Autodesk Inventor part; units mm, degrees
ref_plane "YZ Plane" through (0, 0, 0) normal (1, 0, 0) x (0, 1, 0)
ref_plane "XZ Plane" through (0, 0, 0) normal (0, 1, 0) x (-1, 0, 0)
ref_plane "XY Plane" through (0, 0, 0) normal (0, 0, 1) x (1, 0, 0)
sketch "Sketch1" plane through (0, 0, 0) normal (0, 1, 0) x (-1, 0, 0)
  line L0 (-10, 14) -> (-10, -14)
  line L1 (-7.5, -16.5) -> (7.5, -16.5)
  line L2 (10, -14) -> (10, 14)
  line L3 (7.5, 16.5) -> (-7.5, 16.5)
  line L4 (-10, 16.5) -> (10, -16.5) construction
  line L5 (-10, -16.5) -> (10, 16.5) construction
  arc A0 (10, 14) -> (7.5, 16.5) centre (7.5, 14) ccw
  arc A1 (7.5, -16.5) -> (10, -14) centre (7.5, -14) ccw
  arc A2 (-10, -14) -> (-7.5, -16.5) centre (-7.5, -14) ccw
  arc A3 (-7.5, 16.5) -> (-10, 14) centre (-7.5, 14) ccw
  circle A4 centre (7.5, 14) radius 1.25
  circle A5 centre (-7.5, 14) radius 1.25
  circle A6 centre (-7.5, -14) radius 1.25
  circle A7 centre (7.5, -14) radius 1.25
  point P0 (0, 0)
  dimension "d0" = 33
  dimension "d1" = 20
  dimension "d2" = 2.5
  dimension "d3" = 2.5
  dimension "d4" = 2.5
  dimension "d5" = 2.5
  dimension "d6" = 2.5
extrude "Extrusion1" add sketch "Sketch1" along normal blind 2
sketch "Sketch2" plane through (0, 2, 0) normal (0, 1, 0) x (1, 0, 0)
  line L0 (-17.9692, -32.7187) -> (-17.5216, 33.3599) construction
  line L1 (-17.5216, 33.3599) -> (32.0714, 33.0239) construction
  line L2 (32.0714, 33.0239) -> (31.6238, -33.0546) construction
  line L3 (31.6238, -33.0546) -> (-17.9692, -32.7187) construction
  circle A0 centre (-7.5, 14) radius 1.25
  circle A1 centre (7.5, 14) radius 1.25
  circle A2 centre (7.5, -14) radius 1.25
  circle A3 centre (-7.5, -14) radius 1.25
  line L4 (-10, 14) -> (-10, -14)
  arc A4 (-10, -14) -> (-7.5, -16.5) centre (-7.5, -14) ccw
  line L5 (-7.5, -16.5) -> (7.5, -16.5)
  arc A5 (7.5, -16.5) -> (10, -14) centre (7.5, -14) ccw
  line L6 (10, -14) -> (10, 14)
  arc A6 (10, 14) -> (7.5, 16.5) centre (7.5, 14) ccw
  line L7 (7.5, 16.5) -> (-7.5, 16.5)
  arc A7 (-7.5, 16.5) -> (-10, 14) centre (-7.5, 14) ccw
  point P0 (0, 0)
decal "Decal1"
sketch "Sketch3" plane through (0, 0, 0) normal (0, -1, 0) x (1, 0, 0)
  circle A0 centre (-7.5, -14) radius 1.25
  circle A1 centre (7.5, -14) radius 1.25
  circle A2 centre (7.5, 14) radius 1.25
  circle A3 centre (-7.5, 14) radius 1.25
  line L0 (-10, 14) -> (-10, -14)
  arc A4 (-10, -14) -> (-7.5, -16.5) centre (-7.5, -14) ccw
  line L1 (-7.5, -16.5) -> (7.5, -16.5)
  arc A5 (7.5, -16.5) -> (10, -14) centre (7.5, -14) ccw
  line L2 (10, -14) -> (10, 14)
  arc A6 (10, 14) -> (7.5, 16.5) centre (7.5, 14) ccw
  line L3 (7.5, 16.5) -> (-7.5, 16.5)
  arc A7 (-7.5, 16.5) -> (-10, 14) centre (-7.5, 14) ccw
  line L4 (-25.6164, -20.5771) -> (-25.6164, 49.1548) construction
  line L5 (-25.6164, 49.1548) -> (26.7185, 49.1548) construction
  line L6 (26.7185, 49.1548) -> (26.7185, -20.5771) construction
  line L7 (26.7185, -20.5771) -> (-25.6164, -20.5771) construction
  line L8 (-7.5, 16.5) -> (7.5, 16.5)
  line L9 (0, 16.5) -> (0, 0)
decal "Decal2"
properties part number "Adafruit Compass"
Could you check a few things on this model? Use its own coordinates, in mm. Give positions to 0.01 mm unless a question says otherwise; leave off trailing zeros. Write each loop counter-clockwise with the first axis right and the second up, starting at its lowest first coordinate (ties: lowest second). Pieces come first, ordered by that corner, then holes. Notation, with made-up numbers: (31.5, 83.5) -> (53.5, 83.5) arc R11 cw to (53.5, 95.5) -> close; hole circle Ø10 at (88.25, 61.25). An arc over 180 degrees is marked (long way). Write each question's results on one line, items separated by ' | '. Start each with the question number.
Q1. Suppose I cut it at A-A, the plane y = 0.7. List the corners of the cut face in (x, z) for me.
Q2. I need wall thicknesses on probe 1 along Z at (x, y) = (-7.5, 0.95); probe 2 along X at (y, z) = (0.95, 14.5); probe 3 along Z at (x, y) = (-6.5, 0.45). Which ranges of each line are inside material? Lowest first, please.
Q3. Suppose I cut it at B-B, the plane x = 7. List the corners of the cut face in (y, z) for me.
Q4. We'd pull the mould along X, two halves only. Please class faces 1 (the face through (7.66, 0.99, -15.24)), 2 (the face through (0, 1, 16.5)), 3 (the face through (-10, 1, 0)): +X half, -X half, draft (parallel to the pull), parting line (faces both ways), or undercut.
Outcome:
1) outline: (-10, -14) arc R2.5 ccw to (-7.5, -16.5) -> (7.5, -16.5) arc R2.5 ccw to (10, -14) -> (10, 14) arc R2.5 ccw to (7.5, 16.5) -> (-7.5, 16.5) arc R2.5 ccw to (-10, 14) -> close; hole circle Ø2.5 at (-7.5, -14); hole circle Ø2.5 at (-7.5, 14); hole circle Ø2.5 at (7.5, -14); hole circle Ø2.5 at (7.5, 14)
2) probe 1: -16.5 to -15.25, -12.75 to 12.75, 15.25 to 16.5 | probe 2: -9.95 to -8.65, -6.35 to 6.35, 8.65 to 9.95 | probe 3: -16.5 to -14.75, -13.25 to 13.25, 14.75 to 16.5
3) outline: (0, -16.5) -> (2, -16.5) -> (2, -15.15) -> (0, -15.15) -> close; (0, -12.85) -> (2, -12.85) -> (2, 12.85) -> (0, 12.85) -> close; (0, 15.15) -> (2, 15.15) -> (2, 16.5) -> (0, 16.5) -> close
4) face 1: undercut | face 2: draft | face 3: -X half
